The model under review builds one solid part; all positions refer to its coordinate system, in mm. Round coordinates to 2 decimals unless told otherwise and drop trailing zeros. Write each loop counter-clockwise with the first axis right and the second up, starting at its lowest first coordinate (ties: lowest second). Pieces come first, ordered by that corner, then holes.
Item 1: Draft analysis for pull direction X (two halves, no side actions). For faces 1 (the face through (1.38, 6.2, -0.78)), 2 (the face through (0.69, 3.1, 0.02)), 3 (the face through (8, 1, 0)), state which applies: +X half, -X half, draft (parallel to the pull), parting line (faces both ways), or undercut.
Item 2: Clearance check with a flat-ended pin moving along its axis: pin 1 Ø3.5 at (x, y) = (0, 30.48) entering from -Z. State where the tip first meets the part, or that it passes through.
Item 3: Add section B-B (x = 0). State how many separate pieces and enclosed holes the cut face has, plus the area to 3 significant figures.
Item 4: To check wall thickness, follow L1, parallel to Y at x = 0, z = 2.3; L2, parallel to Y at x = 0, z = 0.05 (1 decimal); L3, parallel to Y at x = 0, z = -0.8 (3 decimals). State the ranges of each line that lie inside material, in increasing order.
Item 5: Add section D-D (y = 15.24). Give the boundary of the cut face in (x, z).
Autodesk Inventor part; units mm, degrees
ref_plane "YZ Plane" through (0, 0, 0) normal (1, 0, 0) x (0, 1, 0)
ref_plane "XZ Plane" through (0, 0, 0) normal (0, 1, 0) x (-1, 0, 0)
ref_plane "XY Plane" through (0, 0, 0) normal (0, 0, 1) x (1, 0, 0)
sketch "Sketch1" plane through (0, 0, 0) normal (0, 0, 1) x (1, 0, 0)
  circle A0 centre (0, 0) radius 38.1
  dimension "d0" = 76.2
extrude "Extrusion1" add sketch "Sketch1" along normal blind 2.54
sketch "Sketch3" plane through (0, 0, 0) normal (0, 0, -1) x (-1, 0, 0)
  circle A0 centre (0, 0) radius 3.175
  circle A1 centre (0, 0) radius 6.35
  circle A2 centre (0, 0) radius 2.3813
  dimension "d4" = 6.35
  dimension "d5" = 12.7
  dimension "d6" = 4.7625
extrude "Extrusion2" cut sketch "Sketch3" against normal blind 25.4 contours A2
extrude "Extrusion3" cut sketch "Sketch3" against normal blind 1.5875 contours A0
extrude "Extrusion4" add sketch "Sketch3" along normal blind 1.5875 contours A1
sketch "Sketch4" plane through (0, 0, 2.54) normal (0, 0, 1) x (1, 0, 0)
  line L0 (0, 0) -> (0, 30.48)
  circle A0 centre (0, 30.48) radius 1.5875
  circle A1 centre (-26.3965, 15.24) radius 1.5875
  circle A2 centre (-26.3965, -15.24) radius 1.5875
  circle A3 centre (0, -30.48) radius 1.5875
  circle A4 centre (26.3965, -15.24) radius 1.5875
  circle A5 centre (26.3965, 15.24) radius 1.5875
  dimension "d13" = 30.48
  dimension "d14" = 3.175
  dimension "d17" = 360
extrude "Extrusion5" cut sketch "Sketch4" against normal blind 25.4
properties part number "SpoolEndFrontSide"
Numbers:
1. face 1: parting line
1. face 2: undercut
1. face 3: draft
2. pin 1: stops at z = 0
3. separate pieces: 4
3. enclosed holes: 0
3. area: 173 mm2
4. L1: y = -38.1 to -32.07, -28.89 to -2.38, 2.38 to 28.89, 32.07 to 38.1
4. L2: y = -38.1 to -32.1, -28.9 to -3.2, 3.2 to 28.9, 32.1 to 38.1
4. L3: y = -6.35 to -3.175, 3.175 to 6.35
5. outline: (-34.92, 0) - (-27.98, 0) - (-27.98, 2.54) - (-34.92, 2.54) - close; (-24.81, 0) - (24.81, 0) - (24.81, 2.54) - (-24.81, 2.54) - close; (27.98, 0) - (34.92, 0) - (34.92, 2.54) - (27.98, 2.54) - close
